Part model, mm, in its own coordinate system. Face numbers are marked on the shaded views. A direction names the side the tool comes from. Give positions to 0.01 mm unless a question says otherwise; leave off trailing zeros. Order: outer loops, then holes, each group sorted by start corner. A loop starts at its lowest first (then second) coordinate and runs counter-clockwise, first axis right, second up. Notation, with made-up numbers: (76, 25.5) - (89, 25.5) arc R18 cw to (89, 45.5) - close; hole circle Ø7 at (70, 57). An arc over 180 degrees is marked (long way). Use one line per item in the form item = value. Start each with the question number.
1. Pull direction Y, two halves, no side cores. Call the marked faces 3, 4 and 5: +Y half, -Y half, draft (parallel to the pull), parting line (faces both ways), or undercut.
2. Tool access for the marked faces 1 and 2: list every direction of +Z, -Z, +X, -X, +Y, -Y with a clear straight run to the whole face (end or side of a thin tool).
3. Band-saw the part on A-A, the plane x = 0. List the corners of the cut face in (y, z), plus the area to 3 significant figures.
4. Band-saw the part on D-D, the plane y = 2. List the corners of the cut face in (x, z).
5. Band-saw the part on C-C, the plane y = 11. List the corners of the cut face in (x, z).
6. Band-saw the part on B-B, the plane z = 0. List the corners of the cut face in (x, y), plus the area to 3 significant figures.
7. Pin check, flat tips, straight feed: P1, Ø8, axis at x = -14.5, y = 2, coming from the +Z side; P2, Ø15, axis at x = 0, z = 0, coming from the +Y side; P3, Ø4, axis at y = 9, z = 10.5, coming from the -X side; P4, Ø4, axis at y = 9.5, z = 10, coming from the +X side. Stop position of each tip, or through.
8. Drill centre lines: line 1 (Z direction, x = 0, y = 8.25); line 2 (Y direction, x = -18.5, z = 35); line 3 (Y direction, x = 28.5, z = 16). Where is each one in solid material? Low to high.
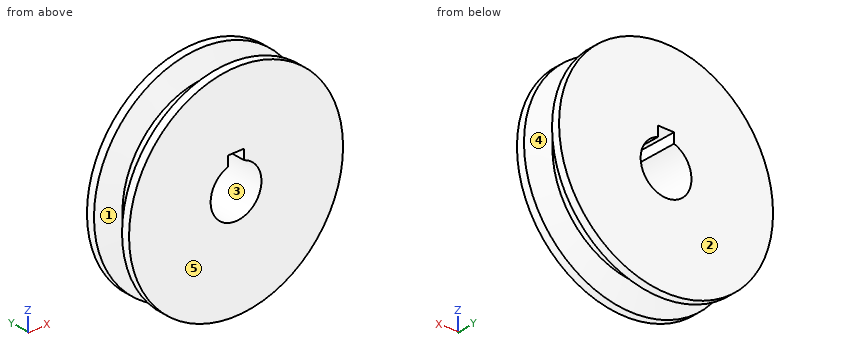
from build123d import *

# Parameters (mm, degrees)
F2_W     = 6
F2_H     = 9.412618
F3_DEPTH = 25


with BuildPart() as f1:
    # F0 (on Top) → F1 (revolve)
    with BuildSketch(Plane.XY):
        Polygon((-40, 0), (-9.5, 0), (-9.5, 18), (-40, 18), (-40, 15), (-32, 12), (-32, 6), (-40, 3), align=None)
    revolve(axis=Axis((0, 10.892909, 0), (0, 1, 0)))

    # F2 (on face) → F3 (cut)
    with BuildSketch(Plane(origin=(0, 18, 0), x_dir=(-1, 0, 0), z_dir=(0, 1, 0))):
        with Locations((0, 7.993691)):
            Rectangle(F2_W, F2_H)
    extrude(amount=-F3_DEPTH, mode=Mode.SUBTRACT)


solid = f1.part
From the geometry:
q1.face_3 = draft
q1.face_4 = undercut
q1.face_5 = -Y half
q2.face_1 = none
q2.face_2 = +Z, -Z, +X, -X, +Y
q3.outline = (0, -40) - (3, -40) - (6, -32) - (12, -32) - (15, -40) - (18, -40) - (18, -9.5) - (0, -9.5) - close; (0, 12.7) - (18, 12.7) - (18, 40) - (15, 40) - (12, 32) - (6, 32) - (3, 40) - (0, 40) - close
q3.area = 896 mm²
q4.outline = circle Ø80 at (0, 0); hole (-3, 9.01) arc R9.5 ccw (long way) to (3, 9.01) - (3, 12.7) - (-3, 12.7) - close
q5.outline = circle Ø64 at (0, 0); hole (-3, 9.01) arc R9.5 ccw (long way) to (3, 9.01) - (3, 12.7) - (-3, 12.7) - close
q6.outline = (-40, 0) - (-9.5, 0) - (-9.5, 18) - (-40, 18) - (-40, 15) - (-32, 12) - (-32, 6) - (-40, 3) - close; (9.5, 0) - (40, 0) - (40, 3) - (32, 6) - (32, 12) - (40, 15) - (40, 18) - (9.5, 18) - close
q6.area = 954 mm²
q7.P1 = 38.6
q7.P2 = through
q7.P3 = -30.85
q7.P4 = 30.98
q8.line_1 = -32 to -9.5, 12.7 to 32
q8.line_2 = 0 to 3.15, 14.85 to 18
q8.line_3 = 0 to 5.74, 12.26 to 18
